Autodesk Inventor part; units mm, degrees
ref_plane "YZ Plane" through (0, 0, 0) normal (1, 0, 0) x (0, 1, 0)
ref_plane "XZ Plane" through (0, 0, 0) normal (0, 1, 0) x (-1, 0, 0)
ref_plane "XY Plane" through (0, 0, 0) normal (0, 0, 1) x (1, 0, 0)
sketch "Skizze1" plane through (0, 0, 0) normal (0, 0, 1) x (1, 0, 0)
  circle A0 centre (0, 0) radius 2
  circle A1 centre (0, 0) radius 4
  circle A2 centre (0, 0) radius 2.4
  circle A3 centre (0, 0) radius 3.6
  dimension "d0" = 4
  dimension "d1" = 8
  dimension "d3" = 0.4
  dimension "d4" = 0.4
extrude "Extrusion1" add sketch "Skizze1" along normal mid plane 2.8 contours A3
extrude "Extrusion2" add sketch "Skizze1" along normal mid plane 3
properties part number "Kugellager 8 x 4 x 3"
Read the model definition and answer for the solid it produces. Units are mm, in the model's axes. Round coordinates to 2 decimals unless told otherwise and drop trailing zeros. Write each loop counter-clockwise with the first axis right and the second up, starting at its lowest first coordinate (ties: lowest second). Pieces come first, ordered by that corner, then holes. Notation, with made-up numbers: M -36,1 L 20,1 A22 cw 20,35 Z; hole C 16.25,-12.75 d4. An arc over 180 degrees is marked long. Use a Markdown table: item, result.
1) A flat-ended cylindrical pin translates along its axis: pin 1 (3.5 mm diameter, centred on x = 0, y = 0, fed in from +Z). Find the tip coordinate at first contact, or state that the pin passes through.
Answers follow:
| item | result |
|---|---|
| pin 1 | passes through |
2) For a pull along Y with two mould halves and no side action, classify faces 1 (the cylindrical face through (0, -2, 0)), 2 (the cylindrical face through (-0.867, 3.905, -0.021)), 3 (the flat face through (-1, 2, 1.5)) as pulls with the +Y half, pulls with the -Y half, needs draft (parallel to the pull), parting line crosses it, or undercut.
Answers follow:
| item | result |
|---|---|
| face 1 | undercut |
| face 2 | parting line crosses it |
| face 3 | needs draft |
3) The part is cut by section C-C (z = 0.3). Write down the section's boundary in (x, y).
Answers follow:
| item | result |
|---|---|
| outline | C 0,0 d8; hole C 0,0 d4 |
4) The part is cut by section A-A (y = 0). Write down the section's boundary in (x, z), plus the area to 3 significant figures.
Answers follow:
| item | result |
|---|---|
| outline | M -4,-1.5 L -3.6,-1.5 L -3.6,-1.4 L -2.4,-1.4 L -2.4,-1.5 L -2,-1.5 L -2,1.5 L -2.4,1.5 L -2.4,1.4 L -3.6,1.4 L -3.6,1.5 L -4,1.5 Z; M 2,-1.5 L 2.4,-1.5 L 2.4,-1.4 L 3.6,-1.4 L 3.6,-1.5 L 4,-1.5 L 4,1.5 L 3.6,1.5 L 3.6,1.4 L 2.4,1.4 L 2.4,1.5 L 2,1.5 Z |
| area | 11.5 mm2 |
5) The part is cut by section D-D (x = -2.25). Write down the section's boundary in (y, z), plus the area to 3 significant figures.
Answers follow:
| item | result |
|---|---|
| outline | M -3.31,-1.5 L -2.81,-1.5 L -2.81,-1.4 L -0.84,-1.4 L -0.84,-1.5 L 0.84,-1.5 L 0.84,-1.4 L 2.81,-1.4 L 2.81,-1.5 L 3.31,-1.5 L 3.31,1.5 L 2.81,1.5 L 2.81,1.4 L 0.84,1.4 L 0.84,1.5 L -0.84,1.5 L -0.84,1.4 L -2.81,1.4 L -2.81,1.5 L -3.31,1.5 Z |
| area | 19.1 mm2 |
6) Straight lines are drawn through the part: line 1 along Y through (x, z) = (0, -1.45); line 2 along Z through (x, y) = (-2.75, 1.25); line 3 along Y through (x, z) = (1.25, 1.3). For each, find the intervals that lie inside material, in ascending order. Write a range as [from, to].
Answers follow:
| item | result |
|---|---|
| line 1 | y = [-4, -3.6], [-2.4, -2], [2, 2.4], [3.6, 4] |
| line 2 | z = [-1.4, 1.4] |
| line 3 | y = [-3.8, -1.56], [1.56, 3.8] |
